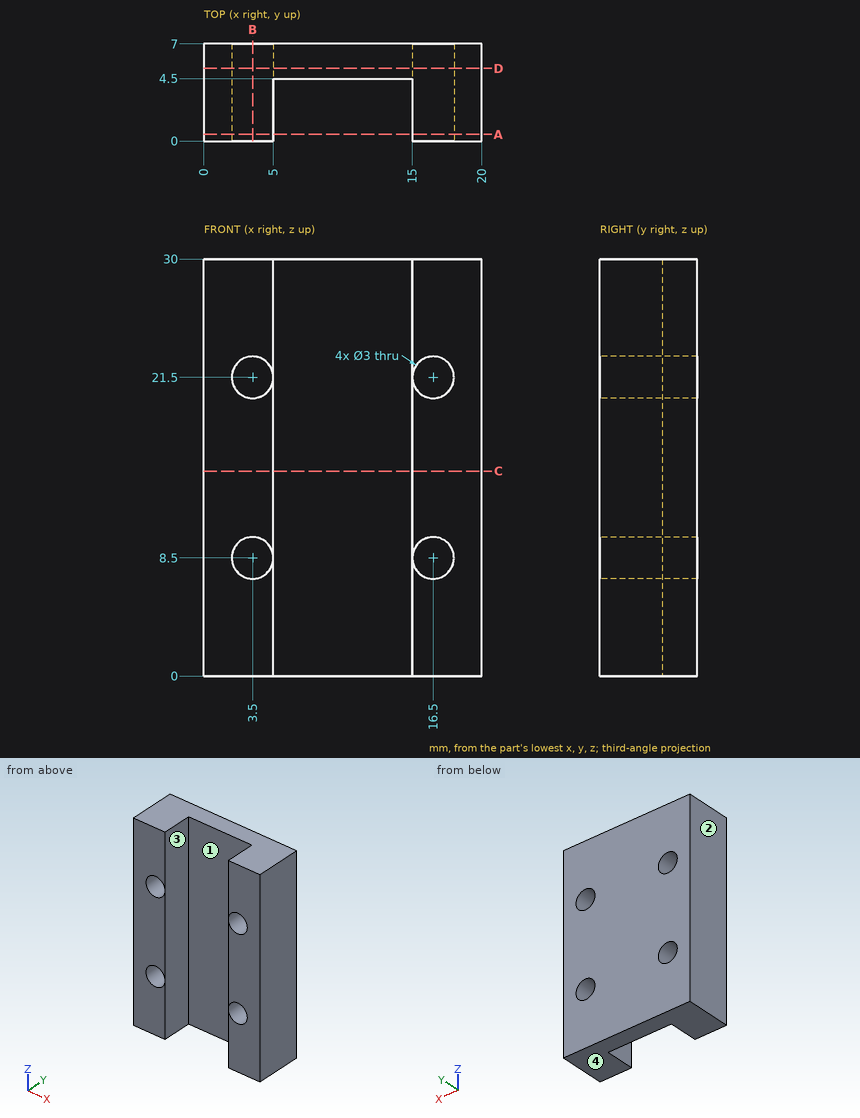
Geometry check sheet. Reference: drawing and pictorial views, mm from the part's lowest x, y, z. Coordinates: 2 decimals unless noted, no trailing zeros. Write each loop counter-clockwise with the first axis right and the second up, starting at its lowest first coordinate (ties: lowest second). Pieces come first, ordered by that corner, then holes.
Item 1: Scan lines: probe 1 along Z at (x, y) = (3.5, 4.75); probe 2 along X at (y, z) = (5.5, 21.5); probe 3 along X at (y, z) = (1.75, 26.5). Record each from-to range of solid material in increasing order.
Numbers:
probe 1: z = 0 to 7, 10 to 20, 23 to 30
probe 2: x = 0 to 2, 5 to 15, 18 to 20
probe 3: x = 0 to 5, 15 to 20
Item 2: Cross-section at D-D on y = 5.25. Record the boundary of the cut face in (x, z), then the cut area to 3 significant figures.
Numbers:
outline: (0, 0) - (20, 0) - (20, 30) - (0, 30) - close; hole circle Ø3 at (3.5, 8.5); hole circle Ø3 at (3.5, 21.5); hole circle Ø3 at (16.5, 8.5); hole circle Ø3 at (16.5, 21.5)
area: 572 mm2
Item 3: Cross-section at C-C on z = 14.75. Record the boundary of the cut face in (x, y), then the cut area to 3 significant figures.
Numbers:
outline: (0, 0) - (5, 0) - (5, 4.5) - (15, 4.5) - (15, 0) - (20, 0) - (20, 7) - (0, 7) - close
area: 95.0 mm2
Item 4: Mould release check, pull along X, two halves, no side actions. Record for the marked faces 1, 2, 3 and 4: released by +X, released by -X, zero draft, split by the parting line, or undercut.
Numbers:
face 1: undercut
face 2: released by -X
face 3: undercut
face 4: zero draft
Item 5: Cross-section at B-B on x = 3.5. Record the boundary of the cut face in (y, z).
Numbers:
outline: (0, 0) - (7, 0) - (7, 7) - (0, 7) - close; (0, 10) - (7, 10) - (7, 20) - (0, 20) - close; (0, 23) - (7, 23) - (7, 30) - (0, 30) - close
Item 6: Cross-section at A-A on y = 0.5. Record the boundary of the cut face in (x, z).
Numbers:
outline: (0, 0) - (5, 0) - (5, 30) - (0, 30) - close; (15, 0) - (20, 0) - (20, 30) - (15, 30) - close; hole circle Ø3 at (3.5, 8.5); hole circle Ø3 at (3.5, 21.5); hole circle Ø3 at (16.5, 8.5); hole circle Ø3 at (16.5, 21.5)
